The model under review builds one solid part; all positions refer to its coordinate system, in mm. A direction names the side the tool comes from. Give positions to 0.01 mm unless a question says otherwise; leave off trailing zeros. Write each loop counter-clockwise with the first axis right and the second up, starting at its lowest first coordinate (ties: lowest second). Pieces come first, ordered by that corner, then holes. Notation, with made-up numbers: (82, 53.25) -> (88, 53.25) arc R22 cw to (88, 86.25) -> close; hole circle Ø1 at (41, -20.75). An arc over 180 degrees is marked (long way). Use CSV: the item, a comma, the result in double quotes.
```python
from build123d import *

# Parameters (mm, degrees)
SKETCH1_W           = 43
SKETCH1_H           = 25
SKETCH1_W_2         = 39
SKETCH1_H_2         = 21
BOSS_EXTRUDE1_DEPTH = 18
SKETCH2_W           = 43
SKETCH2_H           = 25
BOSS_EXTRUDE2_DEPTH = 2
SKETCH3_W           = 43
SKETCH3_H           = 20
CUT_EXTRUDE1_DEPTH  = 2
SKETCH5_W           = 28
SKETCH5_H           = 23
BOSS_EXTRUDE3_DEPTH = 2
SKETCH7_W           = 5
SKETCH7_H           = 2
CUT_EXTRUDE3_DEPTH  = 57.5
BOSS_EXTRUDE4_DEPTH = 2
BOSS_EXTRUDE5_DEPTH = 2
SKETCH18_R          = 1.25
CUT_EXTRUDE4_DEPTH  = 2
FILLET4_R           = 3
FILLET5_R           = 3


with BuildPart() as part:
    # Sketch1 → Boss-Extrude1 (new body)
    with BuildSketch(Plane.XY):
        with Locations((19.5, -10.5)):
            Rectangle(SKETCH1_W, SKETCH1_H)
        with Locations((19.5, -10.5)):
            Rectangle(SKETCH1_W_2, SKETCH1_H_2, mode=Mode.SUBTRACT)
    extrude(amount=BOSS_EXTRUDE1_DEPTH)

    # Sketch2 → Boss-Extrude2 (add)
    with BuildSketch(Plane(origin=(0, 0, 0), x_dir=(-1, 0, 0), z_dir=(0, 0, -1))):
        with Locations((-19.5, -10.5)):
            Rectangle(SKETCH2_W, SKETCH2_H)
    extrude(amount=BOSS_EXTRUDE2_DEPTH)

    # Sketch3 → Cut-Extrude1 (cut)
    with BuildSketch(Plane(origin=(0, 2, 0), x_dir=(1, 0, 0), z_dir=(0, 1, 0))):
        with Locations((19.5, -8)):
            Rectangle(SKETCH3_W, SKETCH3_H)
    extrude(amount=-CUT_EXTRUDE1_DEPTH, mode=Mode.SUBTRACT)

    # Sketch5 → Boss-Extrude3 (add)
    with BuildSketch(Plane.XY.offset(18)):
        with Locations((12, -11.5)):
            Rectangle(SKETCH5_W, SKETCH5_H)
    extrude(amount=BOSS_EXTRUDE3_DEPTH)

    # Sketch7 → Cut-Extrude3 (cut, symmetric)
    with BuildSketch(Plane.ZY.offset(-39)):
        with Locations((9, -3)):
            Rectangle(SKETCH7_W, SKETCH7_H)
    extrude(amount=CUT_EXTRUDE3_DEPTH, both=True, mode=Mode.SUBTRACT)

    # Sketch9 → Boss-Extrude4 (add)
    with BuildSketch(Plane.XY.offset(18)):
        Polygon((26, -21), (39, -21), (39, 0), (41, 0), (41, -23), (26, -23), align=None)
    extrude(amount=BOSS_EXTRUDE4_DEPTH)

    # Sketch14 → Boss-Extrude5 (add)
    with BuildSketch(Plane(origin=(0, 0, 0), x_dir=(1, 0, 0), z_dir=(0, 1, 0))):
        Polygon((26, -18), (26, -20), (-2, -20), (-2, 2), (41, 2), (41, -20), (39, -20), (39, 0), (0, 0), (0, -18), align=None)
    extrude(amount=BOSS_EXTRUDE5_DEPTH)

    # Sketch18 → Cut-Extrude4 (cut)
    with BuildSketch(Plane.XZ.offset(23)):
        with Locations((29.5, 7)):
            Circle(SKETCH18_R)
        with Locations((9.5, 7)):
            Circle(SKETCH18_R)
    extrude(amount=-CUT_EXTRUDE4_DEPTH, mode=Mode.SUBTRACT)

    # Fillet4
    fillet4_edges = [part.edges().sort_by_distance(p)[0] for p in [
        (-2, -10.5, -2),
        (41, -10.5, -2),
        (-2, -10.5, 20),
    ]]
    fillet(fillet4_edges, radius=FILLET4_R)

    # Fillet5
    fillet5_edges = [part.edges().sort_by_distance(p)[0] for p in [
        (41, -10.5, 20),
    ]]
    fillet(fillet5_edges, radius=FILLET5_R)


solid = part.part
```
Q1. Machinability: for faces 1 (the flat face through (40, -3, 6.5)), 2 (the flat face through (0, -10, 9)), 3 (the flat face through (26, -10, 19)), which of the approach directions +Z, -Z, +X, -X, +Y, -Y give a long, thin tool a straight path to every point of the face, cutting with its end or side? Answer none if there is none.
Derived:
face 1,"+X, -X"
face 2,"+Y"
face 3,"+Z, +Y"
Q2. Insertion check: pin 1 (1.5 mm diameter, centred on x = 29.5, z = 7, fed in from +Y); pin 2 (1.6 mm diameter, centred on x = 40, y = -3, fed in from -Z); pin 3 (0.6 mm diameter, centred on y = -10, z = 19.5, fed in from +X); pin 4 (1 mm diameter, centred on x = -0.5, y = -3, fed in from -Z). Each pin has a flat end and moves straight along its axis. Give the tip position at first contact, or say it passes through.
Derived:
pin 1,"passes through"
pin 2,"stops at z = -1.75"
pin 3,"stops at x = 40.04"
pin 4,"stops at z = -1.83"
Q3. Consider section B-B (y = -3.5). Write out the cut boundary in (x, z).
Derived:
outline,"(-2, 1) arc R3 ccw to (1, -2) -> (38, -2) arc R3 ccw to (41, 1) -> (41, 6.5) -> (39, 6.5) -> (39, 0) -> (0, 0) -> (0, 6.5) -> (-2, 6.5) -> close; (-2, 11.5) -> (0, 11.5) -> (0, 18) -> (26, 18) -> (26, 20) -> (1, 20) arc R3 ccw to (-2, 17) -> close; (39, 11.5) -> (41, 11.5) -> (41, 17) arc R3 ccw to (39, 19.83) -> close"
Q4. Consider section C-C (x = 9.5). Write out the cut boundary in (y, z).
Derived:
outline,"(-23, -2) -> (2, -2) -> (2, 0) -> (-21, 0) -> (-21, 5.75) -> (-23, 5.75) -> close; (-23, 8.25) -> (-21, 8.25) -> (-21, 18) -> (2, 18) -> (2, 20) -> (-23, 20) -> close"
Q5. The part is to be moulded in two halves that separate along X. For faces 4 (the cylindrical face through (8.25, -22.01, 7.05)), 5 (the cylindrical face through (-1.1, -10.68, 19.14)), 6 (the cylindrical face through (40.1, -10.68, -1.14)), 7 (the flat face through (13, -10, 18)), say which applies: pulls with the +X half, pulls with the -X half, needs draft (parallel to the pull), parting line crosses it, or undercut.
Derived:
face 4,"undercut"
face 5,"pulls with the -X half"
face 6,"pulls with the +X half"
face 7,"undercut"
Q6. Consider section D-D (y = -18.75). Write out the cut boundary in (x, z).
Derived:
outline,"(-2, 1) arc R3 ccw to (1, -2) -> (38, -2) arc R3 ccw to (41, 1) -> (41, 17) arc R3 ccw to (39, 19.83) -> (39, 0) -> (0, 0) -> (0, 18) -> (26, 18) -> (26, 20) -> (1, 20) arc R3 ccw to (-2, 17) -> close"
Q7. Consider section A-A (z = 8.75). Write out the cut boundary in (x, y), then the cut area to 3 significant figures.
Derived:
outline,"(-2, -23) -> (41, -23) -> (41, -4) -> (39, -4) -> (39, -21) -> (0, -21) -> (0, -4) -> (-2, -4) -> close; (-2, -2) -> (0, -2) -> (0, 2) -> (-2, 2) -> close; (39, -2) -> (41, -2) -> (41, 2) -> (39, 2) -> close"
area,"170 mm2"
Q8. To check wall thickness, follow probe 1 along Z at (x, y) = (9.5, -21.9); probe 2 along X at (y, z) = (-7, 2); probe 3 along Z at (x, y) = (13, -2.75). State the ranges of each line that lie inside material, in increasing order.
Derived:
probe 1,"z = -2 to 5.75, 8.25 to 20"
probe 2,"x = -2 to 0, 39 to 41"
probe 3,"z = -2 to 0, 18 to 20"
